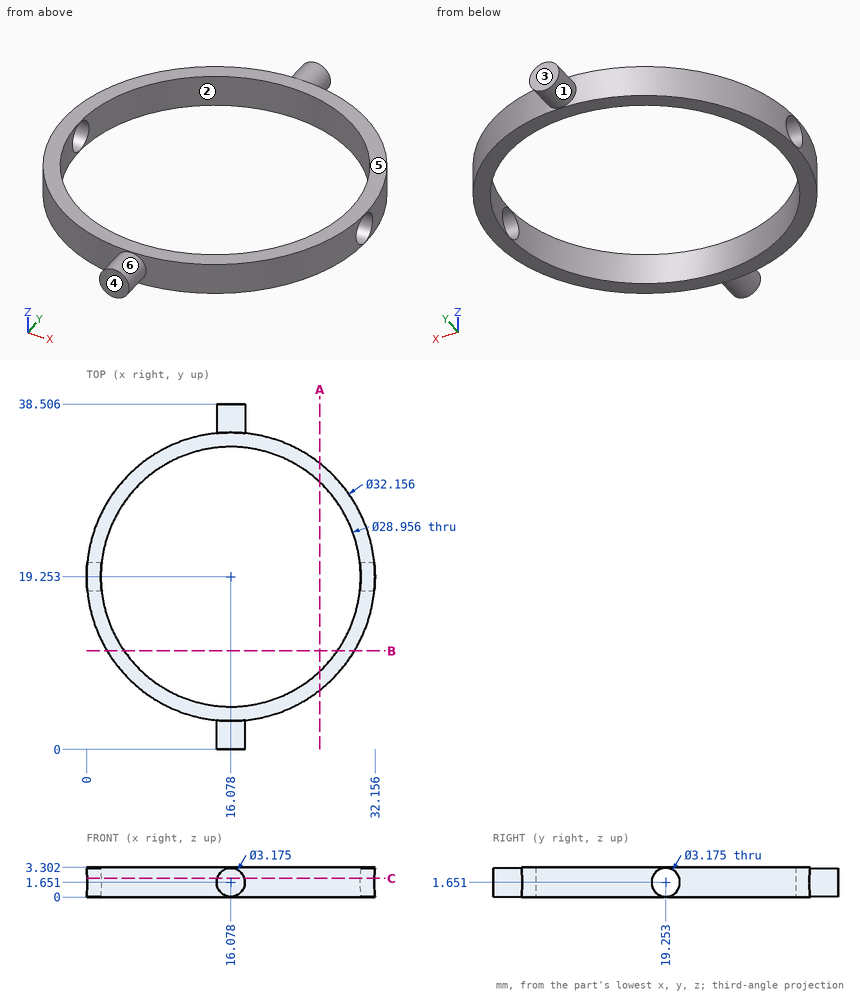
For this review, use the dimensioned drawing (mm, ordinates from the lowest corner) and the shaded views. A direction names the side the tool comes from. Round coordinates to 2 decimals unless told otherwise and drop trailing zeros. Write each loop counter-clockwise with the first axis right and the second up, starting at its lowest first coordinate (ties: lowest second). Pieces come first, ordered by that corner, then holes. Notation, with made-up numbers: (43.25, 64) - (69.25, 64) arc R20 cw to (69.25, 79) - close; hole circle Ø9 at (80.5, 66.5). An arc over 180 degrees is marked (long way). One line per item, written item: value. Start each with the question number.
1. Clearance check with flat-ended pins moving along their axes: P1, Ø1, axis at x = 26, y = 6.5, coming from the -Z side; P2, Ø1.5, axis at y = 9.5, z = 0.5, coming from the -X side. State where each tip first meets the part, or that it passes through.
2. Consider section B-B on y = 11. Write out the cut boundary in (x, z), and give its area (3 significant figures).
3. To check wall thickness, follow L1, parallel to Y at x = 16.5, z = 1.65; L2, parallel to Y at x = 6, z = 2; L3, parallel to X at y = 11, z = 0.95. State the ranges of each line that lie inside material, in increasing order. Write a range as from..to.
4. Consider section C-C on z = 2.1. Write out the cut boundary in (x, y).
5. Consider section A-A on x = 26. Write out the cut boundary in (y, z).
6. Machinability: for the marked faces 5 and 6, which of the approach directions +Z, -Z, +X, -X, +Y, -Y give a long, thin tool a straight path to every point of the face, cutting with its end or side? Answer none if there is none.
7. The part is to be moulded in two halves that separate along Y. For the marked faces 1, 2, 3 and 4, say which applies: released by +Y, released by -Y, zero draft, split by the parting line, or undercut.
Checks:
1. P1: stops at z = 0
1. P2: stops at x = 2.76
2. outline: (2.28, 0) - (4.18, 0) - (4.18, 3.3) - (2.28, 3.3) - close; (27.97, 0) - (29.88, 0) - (29.88, 3.3) - (27.97, 3.3) - close
2. area: 12.6 mm^2
3. L1: y = 0..4.78, 33.72..38.51
3. L2: y = 6.73..8.86, 29.65..31.78
3. L3: x = 2.28..4.18, 27.97..29.88
4. outline: (0.07, 17.73) arc R16.08 ccw to (14.56, 3.25) - (14.56, 0) - (17.6, 0) - (17.6, 3.25) arc R16.08 ccw to (32.08, 17.73) - (30.48, 17.73) arc R14.48 cw to (1.68, 17.73) - close; (0.07, 20.78) - (1.68, 20.78) arc R14.48 cw to (30.48, 20.78) - (32.08, 20.78) arc R16.08 ccw to (17.6, 35.26) - (17.6, 38.51) - (14.56, 38.51) - (14.56, 35.26) arc R16.08 ccw to start
5. outline: (6.6, 0) - (8.71, 0) - (8.71, 3.3) - (6.6, 3.3) - close; (29.8, 0) - (31.9, 0) - (31.9, 3.3) - (29.8, 3.3) - close
6. face 5: +Z, +X, -X, +Y, -Y
6. face 6: -Y
7. face 1: zero draft
7. face 2: undercut
7. face 3: released by +Y
7. face 4: released by -Y
